Build history of the part. All positions in model axes, mm. A direction names the side the tool comes from. Give positions to 0.01 mm unless a question says otherwise; leave off trailing zeros. Order: outer loops, then holes, each group sorted by start corner. A loop starts at its lowest first (then second) coordinate and runs counter-clockwise, first axis right, second up. Notation, with made-up numbers: (-5.5, 16.5) - (16.5, 16.5) arc R14 ccw to (16.5, 38.5) - close; hole circle Ø5 at (-23, 6). An arc over 180 degrees is marked (long way). Write each question's results on one line, items separated by ' | '. Start each with the question number.
1) Cut at D-D on y = 8.75. List the corners of the cut face in (x, z).
2) Cut at A-A on x = 0. List the corners of the cut face in (y, z).
3) Two-plate mould, pull along Y, no slides. Class faces 5 (the face through (-6.7, 7, 1)), 6 (the face through (0, 0, 4)), 7 (the face through (0.1, -6.7, 1.2)): +Y half, -Y half, draft (parallel to the pull), parting line (faces both ways), or undercut.
4) Drill centre lines: line 1 along Y through (x, z) = (1.5, 3); line 2 along Z through (x, y) = (-3.25, -2.5); line 3 along Y through (x, z) = (-2, 3). Where is each one in solid material? Low to high. Write a range as from..to.
5) Cut at B-B on z = 1.25. List the corners of the cut face in (x, y), plus the area to 3 significant figures.
6) Tool access for faces 1 (the face through (0, 19.2, 4)), 2 (the face through (2.6, -3, 4)), 3 (the face through (-2.6, 17, 4)), 4 (the face through (0, -5.2, 4)): list every direction of +Z, -Z, +X, -X, +Y, -Y with a clear straight run to the whole face (end or side of a thin tool).
7) Drop flat-ended pins along their axis: pin 1 Ø1.5 at (y, z) = (16.5, 4) entering from +X; pin 2 Ø3 at (x, y) = (2.5, -0.5) entering from +Z; pin 3 Ø1.5 at (x, z) = (-1, 4) entering from +Y; pin 4 Ø0.9 at (y, z) = (-3, 4.5) entering from -X. Give the stop position or say it passes through.
8) Cut at C-C on y = -3.75. List the corners of the cut face in (x, z).
from build123d import *

# Parameters (mm, degrees)
BOSS_EXTRUDE1_DEPTH = 2.5
SKETCH2_W           = 5.2
SKETCH2_H           = 5.2
BOSS_EXTRUDE2_DEPTH = 4
FILLET1_R           = 1


with BuildPart() as part:
    # Sketch1 → Boss-Extrude1 (new body)
    with BuildSketch(Plane(origin=(0, 0, 0), x_dir=(0, 1, 0), z_dir=(0, 0, 1))):
        with BuildLine():
            Line((0, 6.7), (14, 6.7))
            ThreePointArc((14, 6.7), (20.7, 0), (14, -6.7))
            Line((14, -6.7), (0, -6.7))
            ThreePointArc((0, -6.7), (-6.7, 0), (0, 6.7))
        make_face()
    extrude(amount=BOSS_EXTRUDE1_DEPTH)

    # Sketch2 → Boss-Extrude2 (add)
    with BuildSketch(Plane.XY.offset(2.5)):
        with Locations((0, -2.6)):
            Rectangle(SKETCH2_W, SKETCH2_H)
        with Locations((0, 16.6)):
            Rectangle(SKETCH2_W, SKETCH2_H)
    extrude(amount=BOSS_EXTRUDE2_DEPTH)

    # Fillet1
    fillet1_edges = [part.edges().sort_by_distance(p)[0] for p in [
        (-2.6, 0, 4.5),
        (-2.6, -5.2, 4.5),
        (2.6, -5.2, 4.5),
        (2.6, 0, 4.5),
        (-2.6, -2.6, 6.5),
        (0, -5.2, 6.5),
        (2.6, -2.6, 6.5),
        (0, 0, 6.5),
        (-2.6, 14, 4.5),
        (2.6, 14, 4.5),
        (2.6, 19.2, 4.5),
        (-2.6, 19.2, 4.5),
        (0, 14, 6.5),
        (2.6, 16.6, 6.5),
        (0, 19.2, 6.5),
        (-2.6, 16.6, 6.5),
    ]]
    fillet(fillet1_edges, radius=FILLET1_R)


solid = part.part
Results:
1) outline: (-6.7, 0) - (6.7, 0) - (6.7, 2.5) - (-6.7, 2.5) - close
2) outline: (-6.7, 0) - (20.7, 0) - (20.7, 2.5) - (19.2, 2.5) - (19.2, 5.5) arc R1 ccw to (18.2, 6.5) - (15, 6.5) arc R1 ccw to (14, 5.5) - (14, 2.5) - (0, 2.5) - (0, 5.5) arc R1 ccw to (-1, 6.5) - (-4.2, 6.5) arc R1 ccw to (-5.2, 5.5) - (-5.2, 2.5) - (-6.7, 2.5) - close
3) face 5: draft | face 6: undercut | face 7: -Y half
4) line 1: -5.2..0, 14..19.2 | line 2: 0..2.5 | line 3: -5.12..-0.08, 14.08..19.12
5) outline: (-6.7, 0) arc R6.7 ccw to (6.7, 0) - (6.7, 14) arc R6.7 ccw to (-6.7, 14) - close | area: 329 mm^2
6) face 1: +Z, +X, -X, +Y | face 2: +Z, +X, +Y, -Y | face 3: +Z, -X, +Y, -Y | face 4: +Z, +X, -X, -Y
7) pin 1: x = 2.6 | pin 2: z = 6.5 | pin 3: y = 19.2 | pin 4: x = -2.6
8) outline: (-5.55, 0) - (5.55, 0) - (5.55, 2.5) - (2.6, 2.5) - (2.6, 5.5) arc R1 ccw to (1.6, 6.5) - (-1.6, 6.5) arc R1 ccw to (-2.6, 5.5) - (-2.6, 2.5) - (-5.55, 2.5) - close
